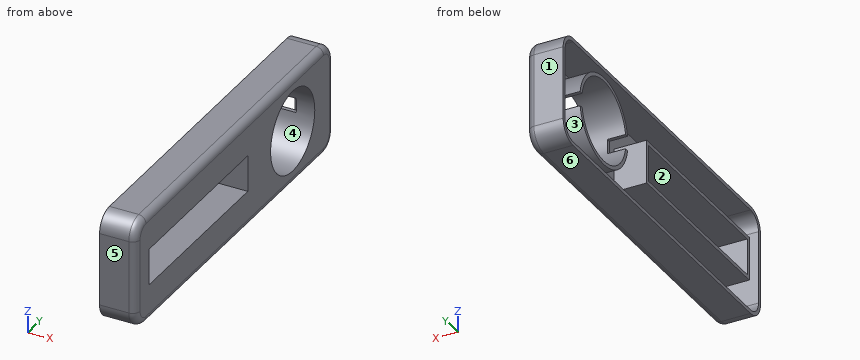
from build123d import *

# Parameters (mm, degrees)
F0_W     = 50
F0_H     = 10
F0_R     = 11.1985350655
F1_DEPTH = 10
F2_T     = -1
F3_R     = 2
F5_DEPTH = 5


with BuildPart() as f1:
    # F0 (on Right) → F1 (new body)
    with BuildSketch(Plane.YZ):
        with BuildLine():
            ThreePointArc((-50, -10), (-48.5355339059, -13.5355339059), (-45, -15))
            Line((-45, -15), (45, -15))
            ThreePointArc((45, -15), (48.5355339059, -13.5355339059), (50, -10))
            Line((50, -10), (50, 10))
            ThreePointArc((50, 10), (48.5355339059, 13.5355339059), (45, 15))
            Line((45, 15), (-45, 15))
            ThreePointArc((-45, 15), (-48.5355339059, 13.5355339059), (-50, 10))
            Line((-50, 10), (-50, -10))
        make_face()
        with Locations((-18.3541104198, 0)):
            Rectangle(F0_W, F0_H, mode=Mode.SUBTRACT)
        with Locations((29.37316522, 0)):
            Circle(F0_R, mode=Mode.SUBTRACT)
    extrude(amount=F1_DEPTH)

    # F2
    f2_openings = [f1.faces().sort_by_distance(p)[0] for p in [
        (0, -47.797293, 12.797293),
    ]]
    offset(amount=F2_T, openings=f2_openings, kind=Kind.INTERSECTION)

    # F3
    f3_edges = [f1.edges().sort_by_distance(p)[0] for p in [
        (10, 0, -15),
        (10, -48.535534, 13.535534),
        (10, -50, 0),
        (10, -48.535534, -13.535534),
        (10, 48.535534, -13.535534),
        (10, 50, 0),
        (10, 48.535534, 13.535534),
        (10, 0, 15),
    ]]
    fillet(f3_edges, radius=F3_R)

    # F4 (on face) → F5 (cut)
    with BuildSketch(Plane(origin=(0, 0, 0), x_dir=(0, -1, 0), z_dir=(-1, 0, 0))):
        with BuildLine():
            Line((-41.4066292992, 2), (-43.37316522, 2))
            Line((-43.37316522, 2), (-43.37316522, -2))
            Line((-43.37316522, -2), (-41.4066292992, -2))
            ThreePointArc((-41.4066292992, -2), (-41.5717002855, 0), (-41.4066292992, 2))
        make_face()
        with BuildLine():
            Line((-40.3916582029, 2), (-41.4066292992, 2))
            ThreePointArc((-41.4066292992, 2), (-41.5717002855, 0), (-41.4066292992, -2))
            Line((-41.4066292992, -2), (-40.3916582029, -2))
            ThreePointArc((-40.3916582029, -2), (-40.5717002855, 0), (-40.3916582029, 2))
        make_face()
        with BuildLine():
            Line((-18.3546722372, 2), (-40.3916582029, 2))
            ThreePointArc((-40.3916582029, 2), (-40.5717002855, 0), (-40.3916582029, -2))
            Line((-40.3916582029, -2), (-18.3546722372, -2))
            ThreePointArc((-18.3546722372, -2), (-18.2197314965, -1.0040437181), (-18.1746301545, 0))
            ThreePointArc((-18.1746301545, 0), (-18.2197314965, 1.0040437181), (-18.3546722372, 2))
        make_face()
        with BuildLine():
            ThreePointArc((-17.1746301545, 0), (-17.2159679428, 1.0034002729), (-17.3397011409, 2))
            Line((-17.3397011409, 2), (-18.3546722372, 2))
            ThreePointArc((-18.3546722372, 2), (-18.2197314965, 1.0040437181), (-18.1746301545, 0))
            ThreePointArc((-18.1746301545, 0), (-18.2197314965, -1.0040437181), (-18.3546722372, -2))
            Line((-18.3546722372, -2), (-17.3397011409, -2))
            ThreePointArc((-17.3397011409, -2), (-17.2159679428, -1.0034002729), (-17.1746301545, 0))
        make_face()
        with BuildLine():
            Line((-15.37316522, 2), (-17.3397011409, 2))
            ThreePointArc((-17.3397011409, 2), (-17.2159679428, 1.0034002729), (-17.1746301545, 0))
            ThreePointArc((-17.1746301545, 0), (-17.2159679428, -1.0034002729), (-17.3397011409, -2))
            Line((-17.3397011409, -2), (-15.37316522, -2))
            Line((-15.37316522, -2), (-15.37316522, 2))
        make_face()
    extrude(amount=-F5_DEPTH, mode=Mode.SUBTRACT)


solid = f1.part
Build history of the part. All positions in model axes, mm. Face numbers are marked on the shaded views. A direction names the side the tool comes from. Round coordinates to 2 decimals unless told otherwise and drop trailing zeros. Loops run counter-clockwise (first coordinate to the right, second up) from the corner with the lowest first, then second, coordinate; pieces in that order, holes last. Notation, with made-up numbers: (53.5, 87.5) -> (104.5, 87.5) arc R17 cw to (104.5, 112.5) -> close; hole circle Ø8 at (-40, -19). An arc over 180 degrees is marked (long way). Use CSV: the item, a comma, the result in double quotes. Start each with the question number.
Q1. Saw through at B-B on y = -27.5. Give the cut face in (x, z), and give its area (3 significant figures).
Q2. Saw through at D-D on y = 11. Give the cut face in (x, z), and give its area (3 significant figures).
Q3. Which spindle directions (+Z, -Z, +X, -X, +Y, -Y) get a long thin tool onto all of the face, cutting with end or side? Do the marked faces 1, 2 and 3. Say none if no direction does.
Q4. Mould opens along Y. For the marked faces 4, 5 and 6 say: +Y half, -Y half, draft (parallel to the pull), parting line (faces both ways), or undercut.
Q5. Saw through at A-A on z = 0. Give the cut face in (x, y), and give its area (3 significant figures).
Q6. Drill centre lines: L1, parallel to Y at x = 3.5, z = 0; L2, parallel to Z at x = 7.75, y = -14.5; L3, parallel to Y at x = 8.25, z = 0. Where is each one in solid material? Low to high.
Q7. Flat gauge pins, fed straight in: pin 1 Ø10 at (y, z) = (38.5, -2) entering from -X; pin 2 Ø5 at (y, z) = (10.5, 7.5) entering from -X; pin 3 Ø1.3 at (y, z) = (17.5, -1) entering from -X. Where does each tip first touch, or does it go through?
Q8. Saw through at C-C on z = 7. Give the cut face in (x, y).
Solutions:
1,outline,"(0, -15) -> (8, -15) arc R2 ccw to (10, -13) -> (10, -5) -> (0, -5) -> (0, -6) -> (9, -6) -> (9, -14) -> (0, -14) -> close; (0, 5) -> (10, 5) -> (10, 13) arc R2 ccw to (8, 15) -> (0, 15) -> (0, 14) -> (9, 14) -> (9, 6) -> (0, 6) -> close"
1,area,"54.3 mm^2"
2,outline,"(0, -15) -> (8, -15) arc R2 ccw to (10, -13) -> (10, 13) arc R2 ccw to (8, 15) -> (0, 15) -> (0, 14) -> (9, 14) -> (9, -14) -> (0, -14) -> close"
2,area,"46.3 mm^2"
3,face 1,"+Z, -Z, +X, -X, +Y"
3,face 2,"+X, -X"
3,face 3,"-X"
4,face 4,"undercut"
4,face 5,"-Y half"
4,face 6,"draft"
5,outline,"(0, -50) -> (8, -50) arc R2 ccw to (10, -48) -> (10, -43.35) -> (0, -43.35) -> (0, -44.35) -> (9, -44.35) -> (9, -49) -> (0, -49) -> close; (0, 6.65) -> (10, 6.65) -> (10, 18.17) -> (5, 18.17) -> (5, 17.17) -> (9, 17.17) -> (9, 7.65) -> (0, 7.65) -> close; (0, 49) -> (9, 49) -> (9, 41.57) -> (5, 41.57) -> (5, 40.57) -> (10, 40.57) -> (10, 48) arc R2 ccw to (8, 50) -> (0, 50) -> close"
5,area,"69.9 mm^2"
6,L1,"y = -50 to -49, -44.35 to -43.35, 6.65 to 7.65, 49 to 50"
6,L2,"z = -15 to -14, -6 to -5, 5 to 6, 14 to 15"
6,L3,"y = -49.98 to -49, -44.35 to -43.35, 6.65 to 7.65, 17.17 to 18.17, 40.57 to 41.57, 49 to 49.98"
7,pin 1,"stops at x = 0"
7,pin 2,"stops at x = 9"
7,pin 3,"stops at x = 5"
8,outline,"(0, -50) -> (8, -50) arc R2 ccw to (10, -48) -> (10, 20.63) -> (0, 20.63) -> (0, 19.38) -> (9, 19.38) -> (9, -49) -> (0, -49) -> close; (0, 38.11) -> (10, 38.11) -> (10, 48) arc R2 ccw to (8, 50) -> (0, 50) -> (0, 49) -> (9, 49) -> (9, 39.36) -> (0, 39.36) -> close"
